Autodesk Inventor part; units mm, degrees
ref_plane "YZ Plane" through (0, 0, 0) normal (1, 0, 0) x (0, 1, 0)
ref_plane "XZ Plane" through (0, 0, 0) normal (0, 1, 0) x (-1, 0, 0)
ref_plane "XY Plane" through (0, 0, 0) normal (0, 0, 1) x (1, 0, 0)
sketch "Sketch1" plane through (0, 0, 0) normal (0, 0, 1) x (1, 0, 0)
  line L0 (11.43, -25.4) -> (11.43, -76.2)
  circle A0 centre (6.35, -38.1) radius 2.0955
  circle A1 centre (6.35, -63.5) radius 2.0955
  line L1 (11.43, -76.2) -> (11.43, -88.9)
  line L2 (11.43, -25.4) -> (11.43, -12.7)
  circle A2 centre (6.35, -12.7) radius 2.0955
  circle A3 centre (6.35, -88.9) radius 2.0955
  line L3 (6.35, -38.1) -> (6.35, -63.5) construction
  line L4 (6.35, -50.8) -> (8.4455, -50.8) construction
  line L5 (6.35, -7.62) -> (-1.2208, -7.62) construction
  line L6 (-1.2208, -7.62) -> (-21.1455, -14.7955) construction
  line L7 (-21.1455, -14.7955) -> (-24.8856, -42.1223) construction
  line L8 (-24.8856, -42.1223) -> (-24.8856, -50.8) construction
  spline S0 degree 4 poles (6.35, -7.62) (-1.2208, -7.62) (-21.1455, -14.7955) (-24.8856, -42.1223) (-24.8856, -50.8) knots 1 1 1 1 1 2 2 2 2 2
  line L9 (6.35, -93.98) -> (-1.2208, -93.98) construction
  line L10 (-1.2208, -93.98) -> (-21.1455, -86.8045) construction
  line L11 (-21.1455, -86.8045) -> (-24.8856, -59.4777) construction
  line L12 (-24.8856, -59.4777) -> (-24.8856, -50.8) construction
  spline S1 degree 4 poles (6.35, -93.98) (-1.2208, -93.98) (-21.1455, -86.8045) (-24.8856, -59.4777) (-24.8856, -50.8) knots 1 1 1 1 1 2 2 2 2 2
  spline S2 degree 4 poles (11.43, -12.7) (11.43, -11.6705) (11.43, -9.6114) (9.4386, -7.8854) (7.3795, -7.62) (6.35, -7.62) knots 0 0 0 0 0 0.5 1 1 1 1 1
  spline S3 degree 4 poles (11.43, -88.9) (11.43, -89.9295) (11.43, -91.9886) (9.4386, -93.7146) (7.3795, -93.98) (6.35, -93.98) knots 0 0 0 0 0 0.5 1 1 1 1 1
  circle A4 centre (-6.35, -25.4) radius 2.1844
  circle A5 centre (-6.35, -76.2) radius 2.1844
  circle A6 centre (0, -44.45) radius 2.1844
  circle A7 centre (0, -57.15) radius 2.1844
  line L13 (-12.7, -30.6578) -> (-12.7, 30.8102)
  circle A8 centre (-19.05, -38.1) radius 2.0955
  circle A9 centre (-19.05, -63.5) radius 2.0955
  point P0 (0, 0)
  dimension "d2" = 4.191
  dimension "d3" = 4.191
  dimension "d4" = 12.7
  dimension "d5" = 4.191
  dimension "d6" = 4.191
  dimension "d9" = 4.191
  dimension "d10" = 6.35
  dimension "d12" = 0
  dimension "d13" = 4.191
  dimension "d14" = 0
  dimension "d15" = 0
extrude "Extrusion2" add sketch "Sketch1" along normal blind 1.524
properties part number "shaft-retainer-v2"
Model file for the job. Use its own axes, mm. Give positions to 0.01 mm unless a question says otherwise; leave off trailing zeros. One line per item, written item: value. Start each with the question number.
1. Probe L1, parallel to Y at x = 6.35, z = 1.05; L2, parallel to Y at x = -19.05, z = 1.15; L3, parallel to Y at x = -6.35, z = 0.75. List the from-to ranges inside material, lowest first. Write a range as from..to.
2. Pull direction Y, two halves, no side cores. Call faces 1 (the flat face through (-3, -50, 0)), 2 (the cylindrical face through (-19.32, -65.58, 0.75)): pulls with the +Y half, pulls with the -Y half, needs draft (parallel to the pull), parting line crosses it, or undercut.
3. Slice it at A-A (x = 0). Give the number of separate pieces and of enclosed holes in the cut face, plus the area to 3 significant figures.
4. Pin check, flat tip, straight feed: pin 1 (3.5 mm diameter, centred on x = 0, y = -57.15, fed in from +Z). Stop position of the tip, or through.
Solution:
1. L1: y = -93.98..-91, -86.8..-65.6, -61.4..-40.2, -36..-14.8, -10.6..-7.62
1. L2: y = -74.2..-65.6, -61.4..-40.2, -36..-27.4
1. L3: y = -89.34..-78.38, -74.02..-27.58, -23.22..-12.26
2. face 1: needs draft
2. face 2: undercut
3. separate pieces: 3
3. enclosed holes: 0
3. area: 114 mm^2
4. pin 1: passes through
